Geometry: final body of the model. Coordinates: model frame, mm. A direction names the side the tool comes from. Give positions to 0.01 mm unless a question says otherwise; leave off trailing zeros. Loops run counter-clockwise (first coordinate to the right, second up) from the corner with the lowest first, then second, coordinate; pieces in that order, holes last. Notation, with made-up numbers: (72.5, 51) -> (80.5, 51) arc R31 ccw to (80.5, 77) -> close; hole circle Ø2 at (-22, 4.25). An arc over 180 degrees is marked (long way). One line per question, with ' | ' between items. Start each with the question number.
Item 1: Section C-C on y = -210. Return loops of the section in (x, z).
Item 2: Pin query (flat end, axial travel): P1, Ø1.5, axis at y = -248, z = 9, coming from the -X side; P2, Ø5, axis at x = -9, y = -105, coming from the +Z side; P3, Ø10, axis at y = -269, z = 46, coming from the -X side. Return the tip coordinate at first contact, or that it passes through.
Item 3: Section A-A on x = 0. Return loops of the section in (y, z), then the cut area to 3 significant figures.
Item 4: Section B-B on z = 47.5. Return loops of the section in (x, y), then the cut area to 3 significant figures.
Item 5: Set-up query: faces 1 (the flat face through (0, -88.716, -3)), 2 (the flat face through (4, 0, 30)). Return all of +Z, -Z, +X, -X, +Y, -Y with unobstructed straight access to the full face (end or side cutting, diameter ignored); none if empty.
Item 6: Section D-D on x = 44. Return loops of the section in (y, z).
Item 7: Material intervals for line 1 along Y through (x, z) = (44.5, 31.5); line 2 along Z through (x, y) = (5, -33.5); line 3 along X through (y, z) = (-106, 5), sorted ascending. Write a range as [from, to].
from build123d import *

# Parameters (mm, degrees)
F0_W     = 98.0357304215
F0_H     = 58.8409267366
F1_DEPTH = 25.4
F2_DEPTH = 67.7178427577
F4_DEPTH = 220.0948596001
F5_R     = 19.1741930287
F6_DEPTH = 130.0617903471
F7_DEPTH = 224.4969811291


with BuildPart() as f1:
    # F0 (on Front) → F1 (new body)
    with BuildSketch(Plane.XZ):
        with Locations((4.3684653938, 29.4204633683)):
            Rectangle(F0_W, F0_H)
    extrude(amount=F1_DEPTH)

    # F2 (add): a face of the model
    f2_faces = [f1.faces().sort_by_distance(p)[0] for p in [
        (4.3684653938, -25.4, 29.4204633683),
    ]]
    extrude(f2_faces, amount=F2_DEPTH)

    # F3 (on face) → F4 (join)
    with BuildSketch(Plane.XZ.offset(93.1178427577)):
        with BuildLine():
            Line((21.0881105967, 0), (-21.0881105967, 0))
            ThreePointArc((-21.0881105967, 0), (0, -7.7051669547), (21.0881105967, 0))
        make_face()
        with BuildLine():
            ThreePointArc((21.0881105967, 0), (29.6628537968, 11.2181038734), (32.7103883216, 25.0052213669))
            ThreePointArc((32.7103883216, 25.0052213669), (-13.7871174935, 54.6680751636), (-21.0881105967, 0))
            Line((-21.0881105967, 0), (21.0881105967, 0))
        make_face()
    extrude(amount=F4_DEPTH)

    # F5 (on face) → F6 (join)
    with BuildSketch(Plane.XZ.offset(313.2127023578)):
        with Locations((0, 25.0052213669)):
            Circle(F5_R)
    extrude(amount=-F6_DEPTH)

    # F7 (add): a face of the model
    f7_faces = [f1.faces().sort_by_distance(p)[0] for p in [
        (0, -313.2127023578, 25.0052213669),
    ]]
    extrude(f7_faces, amount=-F7_DEPTH)


solid = f1.part
Result sheet:
1) outline: circle Ø65.42 at (0, 25.01)
2) P1: stops at x = -28.94 | P2: stops at z = 57.06 | P3: stops at x = -28.53
3) outline: (-313.21, -7.71) -> (-88.72, -7.71) -> (-88.72, 0) -> (0, 0) -> (0, 58.84) -> (-93.12, 58.84) -> (-93.12, 57.72) -> (-313.21, 57.72) -> close | area: 19,900 mm²
4) outline: (-44.65, -93.12) -> (-23.75, -93.12) -> (-23.75, -313.21) -> (23.75, -313.21) -> (23.75, -93.12) -> (53.39, -93.12) -> (53.39, 0) -> (-44.65, 0) -> close | area: 19,600 mm²
5) face 1: -Z, +X, -X, +Y | face 2: +Z, -Z, +X, -X, +Y
6) outline: (-93.12, 0) -> (0, 0) -> (0, 58.84) -> (-93.12, 58.84) -> close
7) line 1: y = [-93.12, 0] | line 2: z = [0, 58.84] | line 3: x = [-25.88, 25.88]
